from build123d import *

# Parameters (mm, degrees)
SKETCH_1_W          = 5.5
SKETCH_1_H          = 3.95
EXTRUDE_1_DEPTH     = 10
CHAMFER_1_SIZE      = 1
SKETCH_2_W          = 8.93689146
SKETCH_2_H          = 16.533425066
CUT_EXTRUDE_1_DEPTH = 5


with BuildPart() as part:
    # ｽｹｯﾁ1 → ﾎﾞｽ - 押し出し1 (new body)
    with BuildSketch(Plane(origin=(0, 0, 0), x_dir=(1, 0, 0), z_dir=(0, 1, 0))):
        Polygon((0, 37.5), (0, 18.75), (23, 18.75), (23, 37.5), (17, 37.5), (11.5, 37.5), (6, 37.5), align=None)
        Polygon((0, 18.75), (0, 0), (6, 0), (11.5, 0), (17, 0), (23, 0), (23, 18.75), align=None)
        with Locations((14.25, -1.975)):
            Rectangle(SKETCH_1_W, SKETCH_1_H)
        with Locations((8.75, -1.975)):
            Rectangle(SKETCH_1_W, SKETCH_1_H)
        with Locations((14.25, 39.475)):
            Rectangle(SKETCH_1_W, SKETCH_1_H)
        with Locations((8.75, 39.475)):
            Rectangle(SKETCH_1_W, SKETCH_1_H)
    extrude(amount=EXTRUDE_1_DEPTH)

    # 面取り1
    chamfer_1_edges = [part.edges().sort_by_distance(p)[0] for p in [
        (6, 5, 3.95),
        (6, 5, 0),
        (0, 5, 0),
        (0, 5, -37.5),
        (6, 5, -37.5),
        (6, 5, -41.45),
        (17, 5, -41.45),
        (17, 5, -37.5),
        (23, 5, -37.5),
        (23, 5, 0),
        (17, 5, 0),
        (17, 5, 3.95),
    ]]
    chamfer(chamfer_1_edges, length=CHAMFER_1_SIZE)

    # ｽｹｯﾁ2 → ｶｯﾄ - 押し出し1 (cut)
    with BuildSketch(Plane(origin=(0, 10, 0), x_dir=(1, 0, 0), z_dir=(0, 1, 0))):
        with Locations((7.03155427, 10.483287467)):
            Rectangle(SKETCH_2_W, SKETCH_2_H)
        with Locations((15.96844573, 10.483287467)):
            Rectangle(SKETCH_2_W, SKETCH_2_H)
        with Locations((15.96844573, 27.016712533)):
            Rectangle(SKETCH_2_W, SKETCH_2_H)
        with Locations((7.03155427, 27.016712533)):
            Rectangle(SKETCH_2_W, SKETCH_2_H)
    extrude(amount=-CUT_EXTRUDE_1_DEPTH, mode=Mode.SUBTRACT)


solid = part.part
Model file for the job. Use its own axes, mm. A direction names the side the tool comes from. Coordinates: 2 decimals unless noted, no trailing zeros. Write each loop counter-clockwise with the first axis right and the second up, starting at its lowest first coordinate (ties: lowest second). Pieces come first, ordered by that corner, then holes. Notation, with made-up numbers: (-1.5, -35.5) -> (8.5, -35.5) arc R36 cw to (8.5, -1.5) -> close; hole circle Ø4 at (77, 85.5). An arc over 180 degrees is marked (long way). One line per item, written item: value. Start each with the question number.
1) Slice it at B-B on z = -22. Write the cut outline in (x, y), then the cut area to 3 significant figures.
2) Slice it at C-C on x = 15. Write the cut outline in (y, z), then the cut area to 3 significant figures.
3) Probe probe 1 along X at (y, z) = (8, -25.5); probe 2 along Z at (x, y) = (9.5, 6); probe 3 along Z at (x, y) = (3.5, 7.75). List the from-to ranges inside material, lowest first.
4) Slice it at A-A on y = 6.75. Write the cut outline in (x, z).
5) Slice it at D-D on y = 1. Write the cut outline in (x, z).
6) Flat gauge pins, fed straight in: pin 1 Ø2 at (x, y) = (20.5, 5) entering from -Z; pin 2 Ø0.6 at (y, z) = (4, -39) entering from -X; pin 3 Ø4.5 at (x, y) = (3, 6.5) entering from +Z. Where does each tip first touch, or does it go through?
7) Pull direction Z, two halves, no side cores. Call faces 5 (the face through (23, 5, -19)), 6 (the face through (16.49, 4.93, -40.96)), 7 (the face through (11, 8, -2.217)): +Z half, -Z half, draft (parallel to the pull), parting line (faces both ways), or undercut.
8) Which spindle directions (+Z, -Z, +X, -X, +Y, -Y) get a long thin tool onto all of the face, cutting with end or side? Do faces 1 (the face through (17, 5, 2)), 2 (the face through (6, 5, 2)), 3 (the face through (0.5, 4.9, -37)), 4 (the face through (11, 5, -19)). Say none if no direction does.
Answers follow:
1. outline: (0, 0) -> (23, 0) -> (23, 10) -> (20.44, 10) -> (20.44, 5) -> (2.56, 5) -> (2.56, 10) -> (0, 10) -> close
1. area: 141 mm2
2. outline: (0, -41.45) -> (10, -41.45) -> (10, -35.28) -> (5, -35.28) -> (5, -2.22) -> (10, -2.22) -> (10, 3.95) -> (0, 3.95) -> close
2. area: 289 mm2
3. probe 1: 0 to 2.56, 20.44 to 23
3. probe 2: -41.45 to -35.28, -2.22 to 3.95
3. probe 3: -37.5 to -35.28, -2.22 to 0
4. outline: (0, -36.5) -> (1, -37.5) -> (5, -37.5) -> (6, -38.5) -> (6, -40.45) -> (7, -41.45) -> (16, -41.45) -> (17, -40.45) -> (17, -38.5) -> (18, -37.5) -> (22, -37.5) -> (23, -36.5) -> (23, -1) -> (22, 0) -> (18, 0) -> (17, 1) -> (17, 2.95) -> (16, 3.95) -> (7, 3.95) -> (6, 2.95) -> (6, 1) -> (5, 0) -> (1, 0) -> (0, -1) -> close; hole (2.56, -35.28) -> (20.44, -35.28) -> (20.44, -2.22) -> (2.56, -2.22) -> close
5. outline: (0, -36.5) -> (1, -37.5) -> (5, -37.5) -> (6, -38.5) -> (6, -40.45) -> (7, -41.45) -> (16, -41.45) -> (17, -40.45) -> (17, -38.5) -> (18, -37.5) -> (22, -37.5) -> (23, -36.5) -> (23, -1) -> (22, 0) -> (18, 0) -> (17, 1) -> (17, 2.95) -> (16, 3.95) -> (7, 3.95) -> (6, 2.95) -> (6, 1) -> (5, 0) -> (1, 0) -> (0, -1) -> close
6. pin 1: z = -37.5
6. pin 2: x = 6
6. pin 3: z = 0.25
7. face 5: draft
7. face 6: -Z half
7. face 7: undercut
8. face 1: +Z, +X, +Y, -Y
8. face 2: +Z, -X, +Y, -Y
8. face 3: -Z, -X, +Y, -Y
8. face 4: +Y
